```python
from build123d import *

# Parameters (mm, degrees)
SKETCH1_R           = 1.595
SKETCH1_R_2         = 1
BOSS_EXTRUDE1_DEPTH = 1


with BuildPart() as part:
    # Sketch1 → Boss-Extrude1 (new body)
    with BuildSketch(Plane.XY):
        with BuildLine():
            Line((12.950297731, 5.25017849), (12.950297731, -9.5))
            Line((12.950297731, -9.5), (17.950297731, -9.5))
            Line((17.950297731, -9.5), (17.950297731, 5.161243048))
            ThreePointArc((17.950297731, 5.161243048), (15.566691032, 11.749406927), (12.950297731, 5.25017849))
        make_face()
        with Locations((15.5, 8)):
            Circle(SKETCH1_R, mode=Mode.SUBTRACT)
        with Locations((15.5, -7)):
            Circle(SKETCH1_R_2, mode=Mode.SUBTRACT)
    extrude(amount=BOSS_EXTRUDE1_DEPTH)


solid = part.part
```
The model under review builds one solid part; all positions refer to its coordinate system, in mm. A direction names the side the tool comes from. Round coordinates to 2 decimals unless told otherwise and drop trailing zeros. Order: outer loops, then holes, each group sorted by start corner. A loop starts at its lowest first (then second) coordinate and runs counter-clockwise, first axis right, second up. Notation, with made-up numbers: (45.5, 58) - (82.5, 58) arc R14 ccw to (82.5, 78) - close; hole circle Ø7 at (41, 76.25). An arc over 180 degrees is marked (long way). Answer in a Markdown table with one row per item.
(1) Machinability: for faces 1 (the face through (17.95, -2.3, 0.5)), 2 (the face through (12.95, -2, 0.5)), 3 (the face through (15, 1, 1)), which of the approach directions +Z, -Z, +X, -X, +Y, -Y give a long, thin tool a straight path to every point of the face, cutting with its end or side? Answer none if there is none.
Result set:
| item | result |
|---|---|
| face 1 | +Z, -Z, +X, -Y |
| face 2 | +Z, -Z, -X, -Y |
| face 3 | +Z, +X, -X, +Y, -Y |
(2) Take a section at B-B on x = 15.5. Write out the cut boundary in (y, z) (3 decimals), plus the area to 3 significant figures.
Result set:
| item | result |
|---|---|
| outline | (-9.5, 0) - (-8, 0) - (-8, 1) - (-9.5, 1) - close; (-6, 0) - (6.405, 0) - (6.405, 1) - (-6, 1) - close; (9.595, 0) - (11.75, 0) - (11.75, 1) - (9.595, 1) - close |
| area | 16.1 mm2 |
(3) Take a section at C-C on z = 0.65. Write out the cut boundary in (x, y) (3 decimals), plus the area to 3 significant figures.
Result set:
| item | result |
|---|---|
| outline | (12.95, -9.5) - (17.95, -9.5) - (17.95, 5.161) arc R3.75 ccw (long way) to (12.95, 5.25) - close; hole circle Ø3.19 at (15.5, 8); hole circle Ø2 at (15.5, -7) |
| area | 103 mm2 |
(4) Mouldability with a two-part tool opening along Y and no side actions: class faces 4 (the face through (15, 1, 0)), 5 (the face through (15.4, -9.5, 0.5)), 6 (the face through (15.154, 6.443, 0.493)), 7 (the face through (16.454, -6.7, 0.493)) as released by +Y, released by -Y, zero draft, split by the parting line, or undercut.
Result set:
| item | result |
|---|---|
| face 4 | zero draft |
| face 5 | released by -Y |
| face 6 | undercut |
| face 7 | undercut |
(5) For line 1 (Y direction, x = 15.5, z = 0.8) (3 decimals); line 2 (Y direction, x = 14.75, z = 0.45); line 3 (X direction, y = -8.5, z = 0.9), list the stretches that pass through material, from the lowest coordinate up. Write a range as from..to.
Result set:
| item | result |
|---|---|
| line 1 | y = -9.5..-8, -6..6.405, 9.595..11.75 |
| line 2 | y = -9.5..-7.66, -6.34..6.59, 9.41..11.67 |
| line 3 | x = 12.95..17.95 |
(6) Take a section at A-A on y = 8. Write out the cut boundary in (x, z) (3 decimals), plus the area to 3 significant figures.
Result set:
| item | result |
|---|---|
| outline | (11.75, 0) - (13.905, 0) - (13.905, 1) - (11.75, 1) - close; (17.095, 0) - (19.25, 0) - (19.25, 1) - (17.095, 1) - close |
| area | 4.31 mm2 |
(7) Clearance check with a flat-ended pin moving along its axis: P1, Ø2.5, axis at x = 15.5, y = 8, coming from the -Z side. State where the tip first meets the part, or that it passes through.
Result set:
| item | result |
|---|---|
| P1 | passes through |
(8) Take a section at D-D on y = -7. Write out the cut boundary in (x, z), plus the area to 3 significant figures.
Result set:
| item | result |
|---|---|
| outline | (12.95, 0) - (14.5, 0) - (14.5, 1) - (12.95, 1) - close; (16.5, 0) - (17.95, 0) - (17.95, 1) - (16.5, 1) - close |
| area | 3.00 mm2 |
